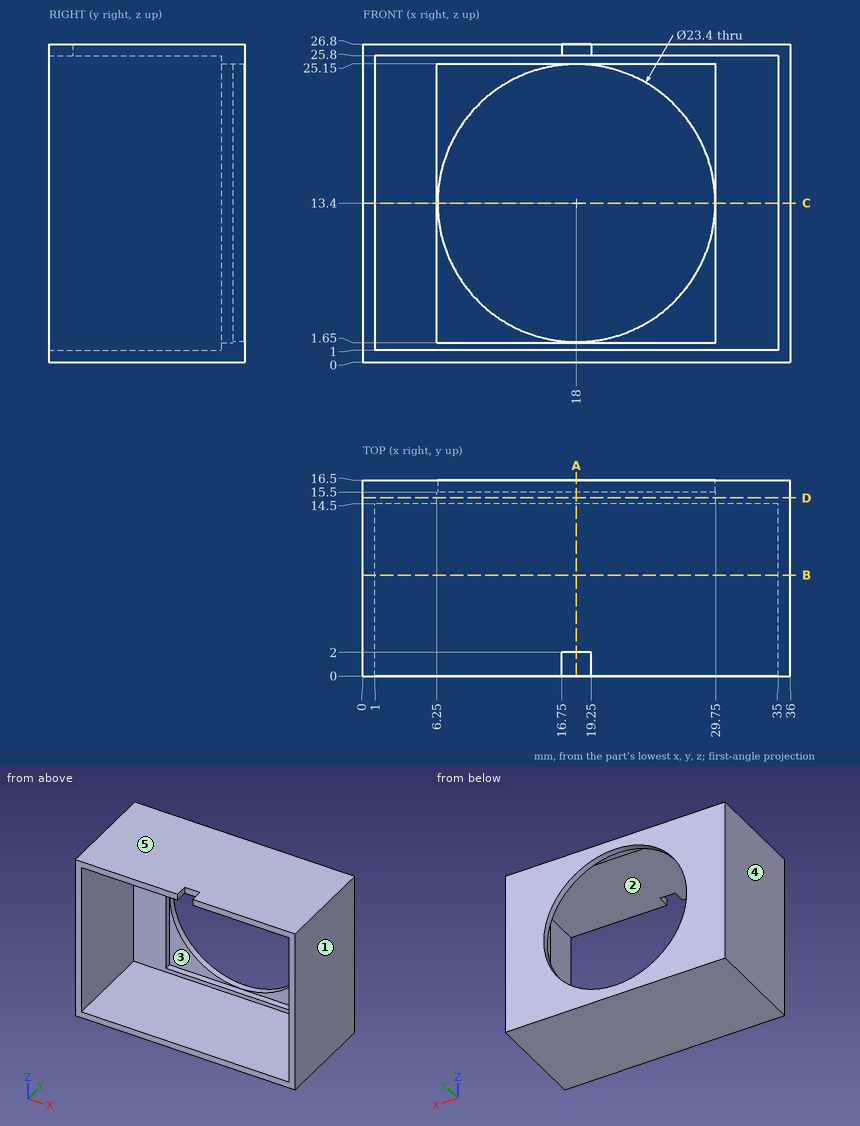
Source: three-view drawing plus pictorial views. Frame: mm from the lowest corner of the part. A direction names the side the tool comes from. Give positions to 0.01 mm unless a question says otherwise; leave off trailing zeros. Write each loop counter-clockwise with the first axis right and the second up, starting at its lowest first coordinate (ties: lowest second). Pieces come first, ordered by that corner, then holes. Notation, with made-up numbers: (71.25, 49) - (122.25, 49) arc R21 cw to (122.25, 70) - close; hole circle Ø3 at (13.5, 19). An arc over 180 degrees is marked (long way). Write item = value, one per line. Start each with the question number.
1. Section query C-C, the plane z = 13.4. Output: boundary loops of the cut face in (x, y), then the cut area to 3 significant figures.
2. Section query D-D, the plane y = 15. Output: boundary loops of the cut face in (x, z), then the cut area to 3 significant figures.
3. Ray query, L1, parallel to Z at x = 27, y = 12.25; L2, parallel to Z at x = 18, y = 16.2; L3, parallel to X at y = 7, z = 17.25. Return the intervals inside material, ascending.
4. First-contact query: pin 1 Ø14 at (x, z) = (18, 13.4) entering from +Y; pin 2 Ø5 at (x, z) = (30.5, 8) entering from -Y; pin 3 Ø1.1 at (x, z) = (17.5, 26) entering from -Y. Flat tips, straight axial feed; report the tip coordinate or a pass-through.
5. Section query A-A, the plane x = 18. Output: boundary loops of the cut face in (y, z), then the cut area to 3 significant figures.
6. Access query for the marked faces 1 and 2. Directions: +Z, -Z, +X, -X, +Y, -Y. A direction counts if a zero-diameter tool reaches every point of the face in a straight line with its end or side. Return the directions, or none.
7. Section query B-B, the plane y = 8.5. Output: boundary loops of the cut face in (x, z).
8. Mould query, pull axis X, two halves, no side actions, for the marked faces 3, 4 and 5. Classes: released by +X, released by -X, zero draft, split by the parting line, or undercut.
Check sheet entries:
q1.outline = (0, 0) - (1, 0) - (1, 14.5) - (6.25, 14.5) - (6.25, 15.5) - (6.3, 15.5) - (6.3, 16.5) - (0, 16.5) - close; (29.7, 15.5) - (29.75, 15.5) - (29.75, 14.5) - (35, 14.5) - (35, 0) - (36, 0) - (36, 16.5) - (29.7, 16.5) - close
q1.area = 54.1 mm2
q2.outline = (0, 0) - (36, 0) - (36, 26.8) - (0, 26.8) - close; hole (6.25, 1.65) - (29.75, 1.65) - (29.75, 25.15) - (6.25, 25.15) - close
q2.area = 413 mm2
q3.L1 = 0 to 1, 25.8 to 26.8
q3.L2 = 0 to 1.7, 25.1 to 26.8
q3.L3 = 0 to 1, 35 to 36
q4.pin_1 = through
q4.pin_2 = 14.5
q4.pin_3 = 2
q5.outline = (0, 0) - (16.5, 0) - (16.5, 1.7) - (15.5, 1.7) - (15.5, 1.65) - (14.5, 1.65) - (14.5, 1) - (0, 1) - close; (2, 25.8) - (14.5, 25.8) - (14.5, 25.15) - (15.5, 25.15) - (15.5, 25.1) - (16.5, 25.1) - (16.5, 26.8) - (2, 26.8) - close
q5.area = 33.7 mm2
q6.face_1 = +Z, -Z, +X, +Y, -Y
q6.face_2 = -Y
q7.outline = (0, 0) - (36, 0) - (36, 26.8) - (0, 26.8) - close; hole (1, 1) - (35, 1) - (35, 25.8) - (1, 25.8) - close
q8.face_3 = undercut
q8.face_4 = released by -X
q8.face_5 = zero draft
